Source: CAD feature listing. Evaluate the final solid. Frame: model axes, mm. A direction names the side the tool comes from. Give positions to 0.01 mm unless a question says otherwise; leave off trailing zeros. Write each loop counter-clockwise with the first axis right and the second up, starting at its lowest first coordinate (ties: lowest second). Pieces come first, ordered by that corner, then holes. Notation, with made-up numbers: (21, -34) - (36, -34) arc R13 cw to (36, -25) - close; hole circle Ø8 at (-28, 76). An arc over 180 degrees is marked (long way). Answer as a JSON object with one key per item and string values. Group by question number.
from build123d import *

# Parameters (mm, degrees)
SKETCH2_W      = 5
SKETCH2_H      = 20
EXTRUDE1_DEPTH = 3.75
SKETCH3_W      = 5
SKETCH3_H      = 13
EXTRUDE2_DEPTH = 2.25
SKETCH4_R      = 1
EXTRUDE3_DEPTH = 3.75


with BuildPart() as part:
    # Sketch2 → Extrude1 (new body)
    with BuildSketch(Plane.XY):
        with Locations((0, -10)):
            Rectangle(SKETCH2_W, SKETCH2_H)
    extrude(amount=EXTRUDE1_DEPTH)

    # Sketch3 → Extrude2 (cut)
    with BuildSketch(Plane(origin=(0, 0, 0), x_dir=(-1, 0, 0), z_dir=(0, 0, -1))):
        with Locations((0, -6.5)):
            Rectangle(SKETCH3_W, SKETCH3_H)
    extrude(amount=-EXTRUDE2_DEPTH, mode=Mode.SUBTRACT)

    # Sketch4 → Extrude3 (cut)
    with BuildSketch(Plane(origin=(0, 0, 0), x_dir=(-1, 0, 0), z_dir=(0, 0, -1))):
        with Locations((0, -18)):
            Circle(SKETCH4_R)
        with Locations((0, -15)):
            Circle(SKETCH4_R)
    extrude(amount=-EXTRUDE3_DEPTH, mode=Mode.SUBTRACT)


solid = part.part
Q1. Ray query, probe 1 along Y at (x, z) = (0, 0.95); probe 2 along Y at (x, z) = (0, 2.65); probe 3 along Y at (x, z) = (-1.65, 0.7). Return the intervals inside material, ascending. Write a range as [from, to].
Q2. Section A-A on y = -15. Return the cut outline in (x, z).
Q3. Section D-D on x = 1.85. Return the cut outline in (y, z).
Q4. Draft query along Y for faces 1 (the flat face through (0, -10, 3.75)), 2 (the flat face through (0, -13, 1)), 3 (the cylindrical face through (0, -16, 2)), 4 (the cylindrical face through (0, -19, 2)). Return one class per face: released by +Y, released by -Y, zero draft, split by the parting line, or undercut.
Q5. Section B-B on x = 0. Return the cut outline in (y, z), then the cut area to 4 significant figures.
Q6. First-contact query: pin 1 Ø3 at (x, y) = (0, -15) entering from -Z; pin 2 Ø1.8 at (x, y) = (0, -18) entering from +Z; pin 3 Ø1.5 at (x, y) = (0.5, -4) entering from -Z; pin 4 Ø0.7 at (x, z) = (-0.5, 0.5) entering from +Y. Flat tips, straight axial feed; report the tip coordinate or a pass-through.
Q7. Section C-C on z = 1.4. Return the cut outline in (x, y), then the cut area to 3 significant figures.
Q8. Reachability of faces 5 (the flat face through (0, -6, 2.25)), 6 (the flat face through (0, 0, 3)) from +Z, -Z, +X, -X, +Y, -Y: full face, straight path, thin tool, end or side. Return the list, or none.
Taken from the geometry:
{
 "1": {"probe 1": "y = [-20, -19], [-17, -16], [-14, -13]", "probe 2": "y = [-20, -19], [-17, -16], [-14, 0]", "probe 3": "y = [-20, -13]"},
 "2": {"outline": "(-2.5, 0) - (-1, 0) - (-1, 3.75) - (-2.5, 3.75) - close; (1, 0) - (2.5, 0) - (2.5, 3.75) - (1, 3.75) - close"},
 "3": {"outline": "(-20, 0) - (-13, 0) - (-13, 2.25) - (0, 2.25) - (0, 3.75) - (-20, 3.75) - close"},
 "4": {"face 1": "zero draft", "face 2": "released by +Y", "face 3": "undercut", "face 4": "undercut"},
 "5": {"outline": "(-20, 0) - (-19, 0) - (-19, 3.75) - (-20, 3.75) - close; (-17, 0) - (-16, 0) - (-16, 3.75) - (-17, 3.75) - close; (-14, 0) - (-13, 0) - (-13, 2.25) - (0, 2.25) - (0, 3.75) - (-14, 3.75) - close", "area": "30.75 mm²"},
 "6": {"pin 1": "stops at z = 0", "pin 2": "passes through", "pin 3": "stops at z = 2.25", "pin 4": "stops at y = -13"},
 "7": {"outline": "(-2.5, -20) - (2.5, -20) - (2.5, -13) - (-2.5, -13) - close; hole circle Ø2 at (0, -18); hole circle Ø2 at (0, -15)", "area": "28.7 mm²"},
 "8": {"face 5": "-Z, +X, -X, +Y", "face 6": "+Z, -Z, +X, -X, +Y"}
}
